```python
from build123d import *

# Parameters (mm, degrees)
SKETCH1_W            = 96.825
SKETCH1_H            = 96.825
BOSS_EXTRUDE1_DEPTH  = 4.7625
FILLET1_R            = 4
M4_CLEARANCE_HOLE1_D = 4.5
M4_CLEARANCE_HOLE2_D = 4.5


with BuildPart() as part:
    # Sketch1 → Boss-Extrude1 (new body, symmetric)
    with BuildSketch(Plane(origin=(0, 0, 0), x_dir=(1, 0, 0), z_dir=(0, 1, 0))):
        Rectangle(SKETCH1_W, SKETCH1_H)
    extrude(amount=BOSS_EXTRUDE1_DEPTH, both=True)

    # Fillet1
    fillet1_edges = [part.edges().sort_by_distance(p)[0] for p in [
        (-48.4125, 0, -48.4125),
        (48.4125, 0, -48.4125),
        (48.4125, 0, 48.4125),
        (-48.4125, 0, 48.4125),
    ]]
    fillet(fillet1_edges, radius=FILLET1_R)

    # M4 Clearance Hole1 (through all)
    with Locations(Plane.ZY.offset(48.4125)):
        with Locations((-30, 0), (30, 0)):
            Hole(M4_CLEARANCE_HOLE1_D / 2)

    # M4 Clearance Hole2 (through all)
    with Locations(Plane(origin=(0, 0, -48.4125), x_dir=(-1, 0, 0), z_dir=(0, 0, -1))):
        with Locations((-30, 0), (30, 0)):
            Hole(M4_CLEARANCE_HOLE2_D / 2)


solid = part.part
```
For this review, take the finished solid that the model builds, in its own axes (mm). Coordinates: 2 decimals unless noted, no trailing zeros. Write each loop counter-clockwise with the first axis right and the second up, starting at its lowest first coordinate (ties: lowest second). Pieces come first, ordered by that corner, then holes. Notation, with made-up numbers: (-2, 21.5) - (47, 21.5) arc R34 cw to (47, 59.5) - close; hole circle Ø9 at (10.5, -28.5). An arc over 180 degrees is marked (long way). Answer in a Markdown table with one row per item. Add a question column.
Q1. For probe 1 along Z at (x, y) = (-10.5, 0); probe 2 along Y at (x, z) = (14, -30); probe 3 along Z at (x, y) = (-18, 1), list the stretches that pass through material, from the lowest coordinate up.
Q2. We need section C-C, the plane y = 0. Count the separate pieces of the cut face and the enclosed holes in it, and give its area (3 significant figures).
Q3. For P1, Ø2.5, axis at y = 0, z = 30, coming from the -X side, flat-tipped, find the tip position at first contact; note if it passes through.
Q4. We need section B-B, the plane z = -34. State the section outline as (x, y) points.
Q5. Draft analysis for pull direction Y (two halves, no side actions). For faces 1 (the flat face through (-1, 0, -48.412)), 2 (the cylindrical face through (0.42, -0.86, -32.08)), 3 (the flat face through (-1, -4.762, -1)), state which applies: +Y half, -Y half, draft (parallel to the pull), parting line (faces both ways), or undercut.
Q6. We need section A-A, the plane x = -42. State the section outline as (y, z) points, and give its area (3 significant figures).
Answer list:
| question | item | result |
|---|---|---|
| 1 | probe 1 | z = -48.41 to -32.25, -27.75 to 27.75, 32.25 to 48.41 |
| 1 | probe 2 | y = -4.76 to -2.25, 2.25 to 4.76 |
| 1 | probe 3 | z = -48.41 to -32.02, -27.98 to 27.98, 32.02 to 48.41 |
| 2 | separate pieces | 9 |
| 2 | enclosed holes | 0 |
| 2 | area | 7,700 mm2 |
| 3 | P1 | passes through |
| 4 | outline | (-48.41, -4.76) - (48.41, -4.76) - (48.41, 4.76) - (-48.41, 4.76) - close; hole circle Ø4.5 at (-30, 0); hole circle Ø4.5 at (30, 0) |
| 5 | face 1 | draft |
| 5 | face 2 | undercut |
| 5 | face 3 | -Y half |
| 6 | outline | (-4.76, -48.41) - (4.76, -48.41) - (4.76, 48.41) - (-4.76, 48.41) - close; hole circle Ø4.5 at (0, -30); hole circle Ø4.5 at (0, 30) |
| 6 | area | 890 mm2 |
